Study the drawing (mm; zero at the part's minimum x, y, z) and answer. Give positions to 0.01 mm unless a question says otherwise; leave off trailing zeros. Write each loop counter-clockwise with the first axis right and the second up, starting at its lowest first coordinate (ties: lowest second). Pieces come first, ordered by that corner, then holes. Notation, with made-up numbers: (13, -30) - (46, -30) arc R34 cw to (46, 4) - close; hole circle Ø8 at (59, 69.5). An arc over 180 degrees is marked (long way). Return JSON: item names as keys, results as strings.
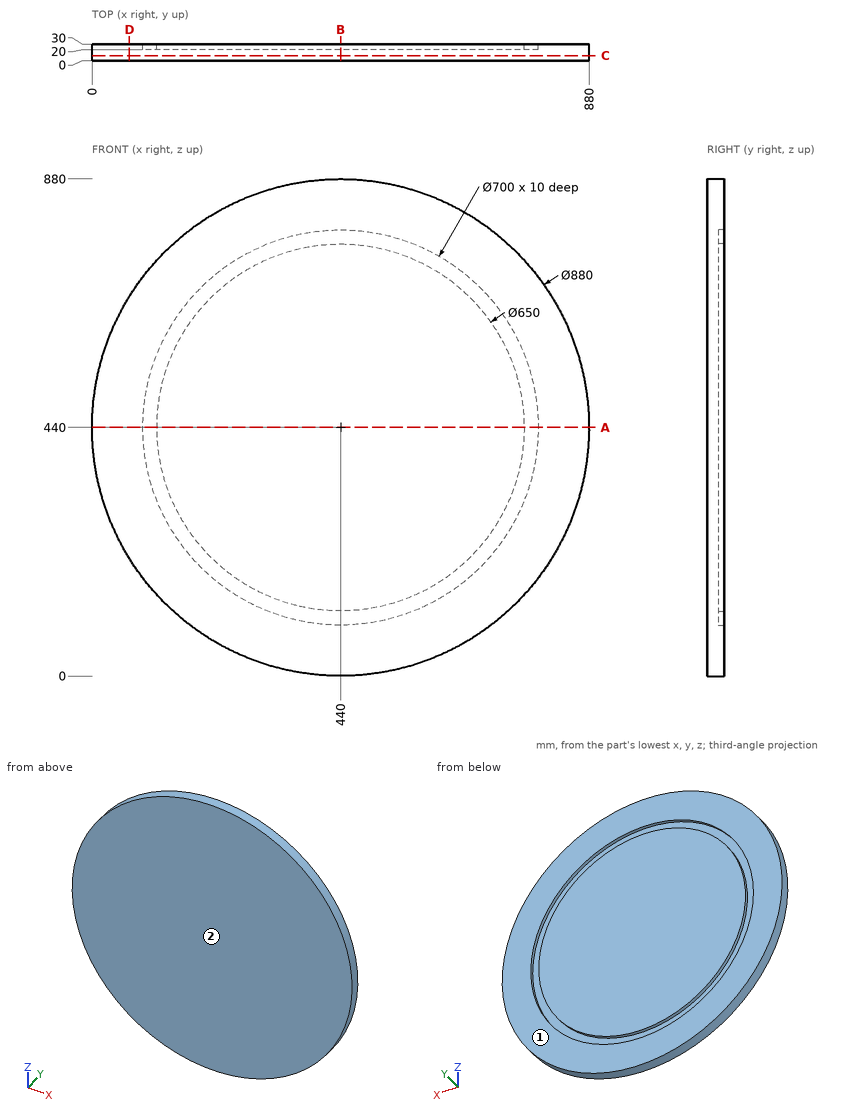
Item 1: A cutting plane is placed at D-D on x = 66. Determine the outline of the cut face in (y, z).
Answer below:
{"outline": "(0, 208.22) - (30, 208.22) - (30, 671.78) - (0, 671.78) - close"}
Item 2: Consider L1, parallel to X at y = 28, z = 440; L2, parallel to Z at x = 447, y = 28; L3, parallel to Z at x = 178.5, y = 28.5. Determine where each line is inside the solid, lowest interval first.
Answer below:
{"L1": "x = 0 to 90, 115 to 765, 790 to 880", "L2": "z = 0.06 to 90.07, 115.08 to 764.92, 789.93 to 879.94", "L3": "z = 86.14 to 207.37, 247.02 to 632.98, 672.63 to 793.86"}
Item 3: A cutting plane is placed at B-B on x = 440. Determine the outline of the cut face in (y, z).
Answer below:
{"outline": "(0, 0) - (30, 0) - (30, 90) - (20, 90) - (20, 115) - (30, 115) - (30, 765) - (20, 765) - (20, 790) - (30, 790) - (30, 880) - (0, 880) - close"}
Item 4: The mould has two halves that part along Y. Classify the marked faces 1 and 2: +Y half, -Y half, draft (parallel to the pull), parting line (faces both ways), or undercut.
Answer below:
{"face 1": "+Y half", "face 2": "-Y half"}
Item 5: A cutting plane is placed at C-C on y = 9.5. Determine the outline of the cut face in (x, z), then the cut area to 3 significant figures.
Answer below:
{"outline": "circle Ø880 at (440, 440)", "area": "608,000 mm²"}
Item 6: Flat-ended cylindrical pins translate along their axes: P1, Ø12, axis at y = 24.5, z = 680, coming from the -X side; P2, Ø4, axis at x = 498, y = 9, coming from the -Z side; P3, Ø3, axis at x = 379, y = 8, coming from the +Z side. Find the tip coordinate at first contact, or state that the pin passes through.
Answer below:
{"P1": "stops at x = 67.38", "P2": "stops at z = 3.58", "P3": "stops at z = 875.96"}
Item 7: A cutting plane is placed at A-A on z = 440. Determine the outline of the cut face in (x, y).
Answer below:
{"outline": "(0, 0) - (880, 0) - (880, 30) - (790, 30) - (790, 20) - (765, 20) - (765, 30) - (115, 30) - (115, 20) - (90, 20) - (90, 30) - (0, 30) - close"}
